from build123d import *

# Parameters (mm, degrees)
F1_DEPTH = 2
F2_R     = 3
F3_DEPTH = 10
F4_R     = 5
F5_DEPTH = 2


with BuildPart() as f1:
    # F0 (on Front) → F1 (new body)
    with BuildSketch(Plane.XZ):
        Polygon((-13.119209, 30.910596), (-38.119209, 30.910596), (-38.119209, 23.410596), (-57.119209, 23.410596), (-57.119209, 13.410596), (-38.119209, 13.410596), (-38.119209, 4.883048), (-13.119209, 4.883048), align=None)
    extrude(amount=F1_DEPTH)

    # F2 (on face) → F3 (join)
    with BuildSketch(Plane.XZ.offset(2)):
        with Locations((-51.215012, 18.444663)):
            Circle(F2_R)
    extrude(amount=F3_DEPTH)

    # F4 (on face) → F5 (join)
    with BuildSketch(Plane.XZ.offset(12)):
        with Locations((-51.215012, 18.444663)):
            Circle(F4_R)
    extrude(amount=F5_DEPTH)


solid = f1.part
Input: part model. Units: mm. Frame: model coordinates. A direction names the side the tool comes from. Give positions to 0.01 mm unless a question says otherwise; leave off trailing zeros. Loops run counter-clockwise (first coordinate to the right, second up) from the corner with the lowest first, then second, coordinate; pieces in that order, holes last. Notation, with made-up numbers: M -5,14.5 L 18,14.5 A11 ccw 18,27.5 Z; hole C 39,46 d8. An arc over 180 degrees is marked long. Use CSV: the item, a comma, the result in double quotes.
(1) Section A-A, the plane x = -47. Return loops of the section in (y, z), plus the area to 3 significant figures.
Outcome:
outline,"M -14,15.76 L -12,15.76 L -12,21.13 L -14,21.13 Z; M -2,13.41 L 0,13.41 L 0,23.41 L -2,23.41 Z"
area,"30.8 mm²"
(2) Material intervals for L1, parallel to Y at x = -33, z = 12.5; L2, parallel to Z at x = -49.5, y = -1.25; L3, parallel to X at y = -9.5, z = 20.25, sorted ascending. Write a range as [from, to].
Outcome:
L1,"y = [-2, 0]"
L2,"z = [13.41, 23.41]"
L3,"x = [-53.61, -48.82]"
(3) Section B-B, the plane z = 16.25. Return loops of the section in (x, y), plus the area to 3 significant figures.
Outcome:
outline,"M -57.12,-2 L -53.26,-2 L -53.26,-12 L -55.71,-12 L -55.71,-14 L -46.72,-14 L -46.72,-12 L -49.17,-12 L -49.17,-2 L -13.12,-2 L -13.12,0 L -57.12,0 Z"
area,"147 mm²"
(4) Pull-direction query (Y, two-part tool) for faces 1 (the face through (-51, -14, 19)), 2 (the face through (-49, -12, 16)), 3 (the face through (-31, 0, 18)), 4 (the face through (-52.299, -12.986, 13.564)); classes: pulls with the +Y half, pulls with the -Y half, needs draft (parallel to the pull), parting line crosses it, or undercut.
Outcome:
face 1,"pulls with the -Y half"
face 2,"undercut"
face 3,"pulls with the +Y half"
face 4,"needs draft"
(5) Section C-C, the plane x = -16.5. Return loops of the section in (y, z), plus the area to 3 significant figures.
Outcome:
outline,"M -2,4.88 L 0,4.88 L 0,30.91 L -2,30.91 Z"
area,"52.1 mm²"
(6) Section D-D, the plane z = 29. Return loops of the section in (x, y).
Outcome:
outline,"M -38.12,-2 L -13.12,-2 L -13.12,0 L -38.12,0 Z"
(7) Set-up query: faces 5 (the face through (-48, -1, 13.411)), 6 (the face through (-26, -1, 4.883)), 7 (the face through (-51.865, -6.93, 15.516)), 8 (the face through (-38.119, -1, 27)). Return all of +Z, -Z, +X, -X, +Y, -Y with unobstructed straight access to the full face (end or side cutting, diameter ignored); none if empty.
Outcome:
face 5,"-Z, -X, +Y, -Y"
face 6,"-Z, +X, -X, +Y, -Y"
face 7,"none"
face 8,"+Z, -X, +Y, -Y"
(8) Pin query (flat end, axial travel): P1, Ø6, axis at x = -34, y = -7, coming from the -Z side; P2, Ø8, axis at x = -45.5, y = -10, coming from the +Z side; P3, Ø2, axis at x = -50, y = -1, coming from the -Z side; P4, Ø0.6, axis at x = -43, y = -1, coming from the +Z side. Return the tip coordinate at first contact, or that it passes through.
Outcome:
P1,"passes through"
P2,"stops at z = 22.91"
P3,"stops at z = 13.41"
P4,"stops at z = 23.41"
